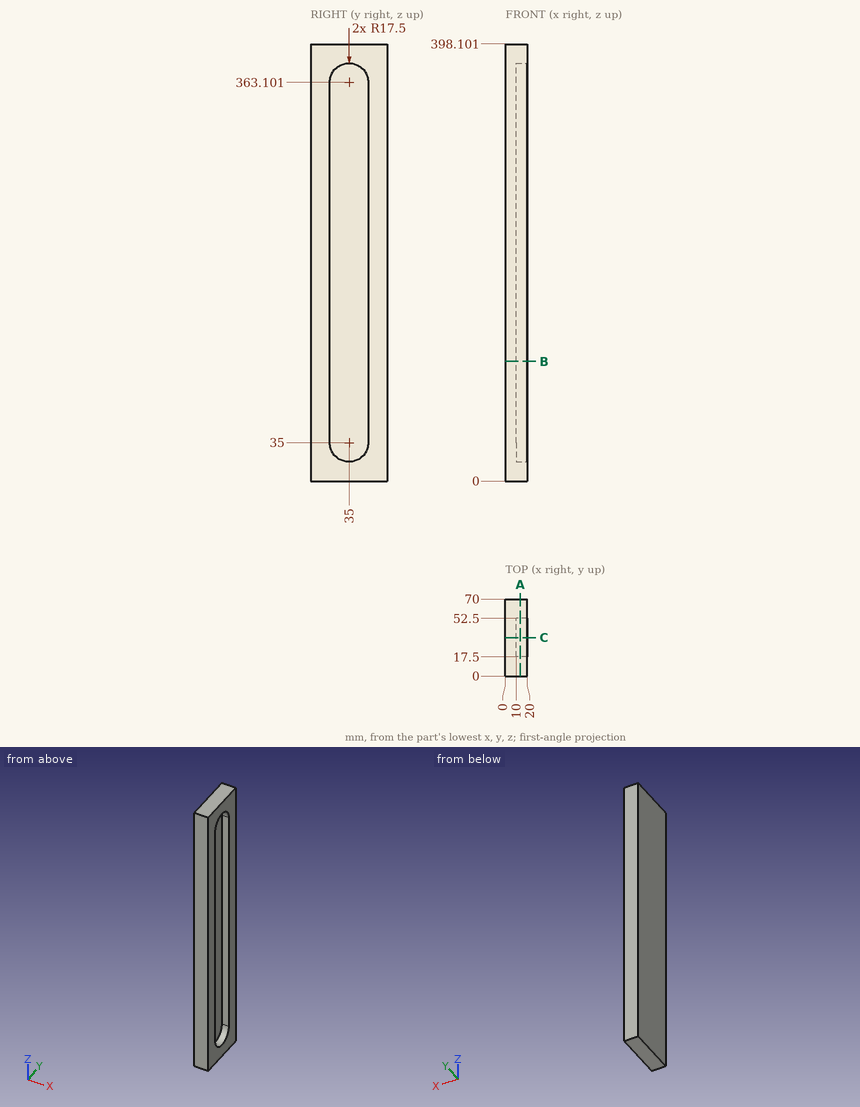
Geometry: see drawing. Coordinates: mm, zero at the bounding-box minimum. Give positions to 0.01 mm unless a question says otherwise; leave off trailing zeros. Loops run counter-clockwise (first coordinate to the right, second up) from the corner with the lowest first, then second, coordinate; pieces in that order, holes last. Notation, with made-up numbers: M -6,1.25 L 21,1.25 A19 ccw 21,38.25 Z; hole C -11.5,-12 d4. An arc over 180 degrees is marked long. Answer as CSV lines item,"result". Start each with the question number.
1. Pin query (flat end, axial travel): P1, Ø3, axis at y = 37.5, z = 236, coming from the -X side; P2, Ø1.5, axis at y = 48.5, z = 192, coming from the +X side. Return the tip coordinate at first contact, or that it passes through.
2. Section A-A on x = 13.5. Return loops of the section in (y, z), plus the area to 3 significant figures.
3. Section B-B on z = 109. Return loops of the section in (x, y), plus the area to 3 significant figures.
4. Section C-C on y = 35. Return loops of the section in (x, z).
5. Line query: L1, parallel to Y at x = 10.5, z = 128; L2, parallel to X at y = 44.5, z = 330; L3, parallel to Z at x = 15.75, y = 29. Output: solid intervals per line, ascending.
Computed values:
1,P1,"stops at x = 0"
1,P2,"stops at x = 10"
2,outline,"M 0,0 L 70,0 L 70,398.1 L 0,398.1 Z; hole M 17.5,35 A17.5 ccw 52.5,35 L 52.5,363.1 A17.5 ccw 17.5,363.1 Z"
2,area,"15,400 mm²"
3,outline,"M 0,0 L 20,0 L 20,17.5 L 10,17.5 L 10,52.5 L 20,52.5 L 20,70 L 0,70 Z"
3,area,"1,050 mm²"
4,outline,"M 0,0 L 20,0 L 20,17.5 L 10,17.5 L 10,380.6 L 20,380.6 L 20,398.1 L 0,398.1 Z"
5,L1,"y = 0 to 17.5, 52.5 to 70"
5,L2,"x = 0 to 10"
5,L3,"z = 0 to 18.56, 379.54 to 398.1"
